from build123d import *

# Parameters (mm, degrees)
F0_W     = 33.256879
F0_H     = 86.122798
F0_W_2   = 23.275094
F0_H_2   = 64.976308
F1_DEPTH = 533.4
F0_R     = 181.374578
F2_DEPTH = 508


with BuildPart() as f1:
    # F0 (on Right) → F1 (new body)
    with BuildSketch(Plane.YZ):
        with Locations((0.07674, 1.116945)):
            Rectangle(F0_W, F0_H)
        with Locations((0.07674, 1.116945)):
            Rectangle(F0_W_2, F0_H_2, mode=Mode.SUBTRACT)
    extrude(amount=F1_DEPTH)

    # F0 (on Right) → F2 (join)
    with BuildSketch(Plane.YZ):
        with Locations((0.07674, 1.116945)):
            Circle(F0_R)
        with Locations((0.07674, 1.116945)):
            Rectangle(F0_W, F0_H, mode=Mode.SUBTRACT)
    extrude(amount=F2_DEPTH)


solid = f1.part
CAD build for the part. Positions are in the model's coordinates, mm. A direction names the side the tool comes from. Round coordinates to 2 decimals unless told otherwise and drop trailing zeros. Loops run counter-clockwise (first coordinate to the right, second up) from the corner with the lowest first, then second, coordinate; pieces in that order, holes last. Notation, with made-up numbers: M 60,31.5 L 118,31.5 A27 cw 118,57.5 Z; hole C 45.25,56.5 d9. An arc over 180 degrees is marked long. One line per question, with ' | ' between items. Start each with the question number.
Item 1: Pin check, flat tips, straight feed: pin 1 Ø2 at (x, z) = (407, 134) entering from -Y; pin 2 Ø4 at (x, y) = (75, -39) entering from +Z; pin 3 Ø2 at (x, y) = (391, -67) entering from -Z. Stop position of each tip, or through.
Item 2: Cut at A-A, the plane z = -7. Write the cut outline in (x, y).
Item 3: Which spindle directions (+Z, -Z, +X, -X, +Y, -Y) get a long thin tool onto all of the face, cutting with end or side? Do faces 1 (the flat face through (521, 0, 44.178)), 2 (the flat face through (521, -16.552, 1)), 3 (the flat face through (521, 16.705, 1)), 4 (the flat face through (263, 0, -31.371)). Say none if no direction does.
Item 4: Two-plate mould, pull along Z, no slides. Class faces 5 (the cylindrical face through (250.444, 97.583, 154.053)), 6 (the flat face through (0, -2, -37)), 7 (the flat face through (263, 11.714, 1)): pulls with the +Z half, pulls with the -Z half, needs draft (parallel to the pull), parting line crosses it, or undercut.
Item 5: Cut at B-B, the plane x = 102. Write the cut outline in (y, z), plus the area to 3 significant figures.
Item 6: Wall check: line 1 (Y direction, x = 325, z = 0); line 2 (Z direction, x = 360.5, y = -5); line 3 (X direction, y = 132, z = -52). Give the ranges that are in metal, low to high.
Item 7: Cut at C-C, the plane y = -106.5. Write the cut outline in (x, z).
Item 8: Cut at D-D, the plane z = -124.5. Write the cut outline in (x, y), plus the area to 3 significant figures.
Responses:
1) pin 1: stops at y = -124.44 | pin 2: stops at z = 178.66 | pin 3: stops at z = -167.79
2) outline: M 0,-181.12 L 508,-181.12 L 508,-16.55 L 533.4,-16.55 L 533.4,-11.56 L 0,-11.56 Z; M 0,11.71 L 533.4,11.71 L 533.4,16.71 L 508,16.71 L 508,181.27 L 0,181.27 Z
3) face 1: +Z, +X, +Y, -Y | face 2: +Z, -Z, +X, -Y | face 3: +Z, -Z, +X, +Y | face 4: +X, -X
4) face 5: parting line crosses it | face 6: needs draft | face 7: undercut
5) outline: C 0.08,1.12 d362.75; hole M -11.56,-31.37 L 11.71,-31.37 L 11.71,33.61 L -11.56,33.61 Z | area: 102,000 mm²
6) line 1: y = -181.29 to -11.56, 11.71 to 181.45 | line 2: z = -180.19 to -31.37, 33.61 to 182.42 | line 3: x = 0 to 508
7) outline: M 0,-145.64 L 508,-145.64 L 508,147.88 L 0,147.88 Z
8) outline: M 0,-130.76 L 508,-130.76 L 508,130.91 L 0,130.91 Z | area: 133,000 mm²
